Source: CAD feature listing. Evaluate the final solid. Frame: model axes, mm. A direction names the side the tool comes from. Round coordinates to 2 decimals unless told otherwise and drop trailing zeros. Loops run counter-clockwise (first coordinate to the right, second up) from the corner with the lowest first, then second, coordinate; pieces in that order, holes last.
(1) Material intervals for probe 1 along Y at (x, z) = (0, 0.3); probe 2 along Y at (x, z) = (4.5, 1.4); probe 3 along X at (y, z) = (5.5, 4.75), sorted ascending.
(2) Section D-D, the plane x = 3.5. Return the cut outline in (y, z).
(3) Section C-C, the plane z = 2.05. Return the cut outline in (x, y).
(4) Section B-B, the plane y = -11.5. Return the cut outline in (x, z).
(5) First-contact query: pin 1 Ø4.5 at (x, y) = (0, -11.5) entering from -Z; pin 2 Ø4.5 at (x, y) = (-12, -1) entering from +Z; pin 3 Ø3 at (x, y) = (0.5, -12.5) entering from +Z; pin 4 Ø3 at (x, y) = (11.5, -0.5) entering from +Z. Flat tips, straight axial feed; report the tip coordinate or a pass-through.
(6) Section A-A, the plane x = 0. Return the cut outline in (y, z).
(7) Set-up query: faces 1 (the flat face through (1.3, 12.9, 1.5)), 2 (the flat face through (-1, -8, 5.5)). Return all of +Z, -Z, +X, -X, +Y, -Y with unobstructed straight access to the full face (end or side cutting, diameter ignored); none if empty.
Autodesk Inventor part; units mm, degrees
ref_plane "YZ Plane" through (0, 0, 0) normal (1, 0, 0) x (0, 1, 0)
ref_plane "XZ Plane" through (0, 0, 0) normal (0, 1, 0) x (-1, 0, 0)
ref_plane "XY Plane" through (0, 0, 0) normal (0, 0, 1) x (1, 0, 0)
sketch "Sketch1" plane through (0, 0, 0) normal (0, 0, 1) x (1, 0, 0)
  circle A0 centre (0, 0) radius 16
  dimension "d0" = 32
extrude "Extrusion1" add sketch "Sketch1" along normal blind 4.5
sketch "Sketch2" plane through (0, 0, 4.5) normal (0, 0, 1) x (1, 0, 0)
  circle A0 centre (0, 0) radius 16
  circle A1 centre (0, 0) radius 8.75
  dimension "d5" = 17.5
extrude "Extrusion2" add sketch "Sketch2" along normal blind 1 contours A1
sketch "Sketch3" plane through (0, 0, 5.5) normal (0, 0, 1) x (1, 0, 0)
  circle A0 centre (0, 0) radius 8.75
  circle A1 centre (0, 0) radius 7.75
  dimension "d10" = 15.5
extrude "Extrusion3" cut sketch "Sketch3" against normal through all contours A1
sketch "Sketch4" plane through (0, 0, 4.5) normal (0, 0, 1) x (1, 0, 0)
  circle A0 centre (0, 0) radius 8.75
  circle A1 centre (0, 11.5) radius 1.75
  dimension "d15" = 11.5
  dimension "d16" = 3.5
extrude "Extrusion4" cut sketch "Sketch4" against normal through all contours A1
pattern_circular "Circular Pattern1" count 4 over 360 about axis through (0, 0, 0) along (0, 0, 1) of "Extrusion4"
sketch "Sketch5" plane through (0, 0, 4.5) normal (0, 0, 1) x (1, 0, 0)
  circle A0 centre (0, 11.5) radius 1.75
  circle A1 centre (0, 0) radius 8.75
  arc A2 (1.044, 8.6875) -> (-1.044, 8.6875) centre (0, 11.5) ccw
  dimension "d22" = 6
extrude "Extrusion5" cut sketch "Sketch5" against normal blind 3 contours A1 A2
sketch "Sketch6" plane through (0, 0, 4.5) normal (0, 0, 1) x (1, 0, 0)
  circle A0 centre (-11.5, 0) radius 1.75
  line L0 (-11.5, 3.1754) -> (-8.75, 1.5877)
  line L1 (-8.75, 1.5877) -> (-8.75, -1.5877)
  line L2 (-8.75, -1.5877) -> (-11.5, -3.1754)
  line L3 (-11.5, -3.1754) -> (-14.25, -1.5877)
  line L4 (-14.25, -1.5877) -> (-14.25, 1.5877)
  line L5 (-14.25, 1.5877) -> (-11.5, 3.1754)
  dimension "d28" = 5.5
extrude "Extrusion6" cut sketch "Sketch6" against normal blind 4
pattern_circular "Circular Pattern2" count 2 over 360 about axis through (0, 0, 0) along (0, 0, 1) of "Extrusion6", "Extrusion5"
properties part number "bearing seat 1"
Output values:
1. probe 1: y = -16 to -13.25, -9.75 to -7.75, 7.75 to 9.75, 13.25 to 16
1. probe 2: y = -15.35 to -6.31, 6.31 to 15.35
1. probe 3: x = -6.81 to -5.46, 5.46 to 6.81
2. outline: (-15.61, 0) - (-6.91, 0) - (-6.91, 5.5) - (-8.02, 5.5) - (-8.02, 4.5) - (-15.61, 4.5) - close; (6.91, 0) - (15.61, 0) - (15.61, 4.5) - (8.02, 4.5) - (8.02, 5.5) - (6.91, 5.5) - close
3. outline: circle Ø32 at (0, 0); hole (-14.25, -1.59) - (-11.5, -3.18) - (-8.75, -1.59) - (-8.75, 1.59) - (-11.5, 3.18) - (-14.25, 1.59) - close; hole circle Ø15.5 at (0, 0); hole (-1.04, -8.69) arc R3 ccw (long way) to (1.04, -8.69) arc R8.75 cw to start; hole (-1.04, 8.69) arc R8.75 cw to (1.04, 8.69) arc R3 ccw (long way) to start; hole (8.75, -1.59) - (11.5, -3.18) - (14.25, -1.59) - (14.25, 1.59) - (11.5, 3.18) - (8.75, 1.59) - close
4. outline: (-11.12, 0) - (-1.75, 0) - (-1.75, 1.5) - (-3, 1.5) - (-3, 4.5) - (-11.12, 4.5) - close; (1.75, 0) - (11.12, 0) - (11.12, 4.5) - (3, 4.5) - (3, 1.5) - (1.75, 1.5) - close
5. pin 1: stops at z = 0
5. pin 2: stops at z = 4.5
5. pin 3: stops at z = 1.5
5. pin 4: stops at z = 0.5
6. outline: (-16, 0) - (-13.25, 0) - (-13.25, 1.5) - (-14.5, 1.5) - (-14.5, 4.5) - (-16, 4.5) - close; (-9.75, 0) - (-7.75, 0) - (-7.75, 5.5) - (-8.75, 5.5) - (-8.75, 1.5) - (-9.75, 1.5) - close; (7.75, 0) - (9.75, 0) - (9.75, 1.5) - (8.75, 1.5) - (8.75, 5.5) - (7.75, 5.5) - close; (13.25, 0) - (16, 0) - (16, 4.5) - (14.5, 4.5) - (14.5, 1.5) - (13.25, 1.5) - close
7. face 1: +Z
7. face 2: +Z, +X, -X, +Y, -Y
